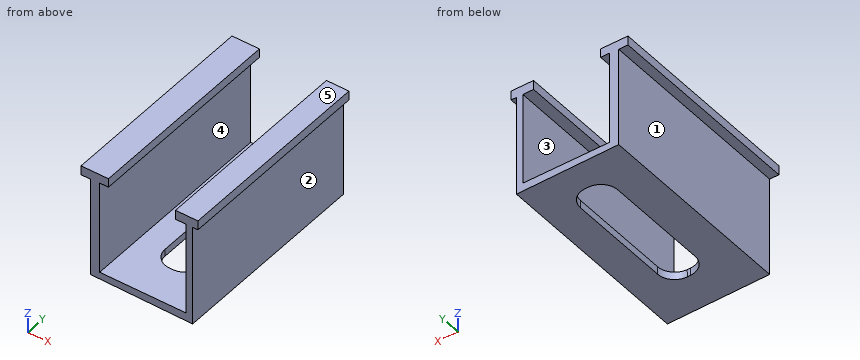
from build123d import *

# Parameters (mm, degrees)
F1_DEPTH = 120
F3_DEPTH = 25
F4_DEPTH = 25


with BuildPart() as f1:
    # F0 (on Front) → F1 (new body)
    with BuildSketch(Plane.XZ):
        Polygon((-31.802535, 29.50009), (-31.802535, 34.680594), (-47.919657, 34.680594), (-47.919657, 29.212285), (-42.451348, 29.212285), (-42.451348, -29.212285), (17.700056, -30.075703), (17.700056, 29.212285), (20.865917, 29.212285), (20.865917, 34.680594), (7.626853, 34.680594), (7.626853, 29.212285), (13.958578, 29.212285), (13.958578, -25.183003), (-36.983039, -25.183003), (-36.983039, 29.50009), align=None)
    extrude(amount=F1_DEPTH)

    # F2 (on face) → F3 (cut)
    with BuildSketch(Plane(origin=(-0.427974, 0, -29.815492), x_dir=(0.999897, 0, -0.014353), z_dir=(-0.014353, 0, -0.999897))):
        with BuildLine():
            Line((-10, 97.833304), (-11.900108, 97.833304))
            ThreePointArc((-11.900108, 97.833304), (-18.971176, 94.904371), (-21.900108, 87.833304))
            Line((-21.900108, 87.833304), (-21.900108, 26.494442))
            ThreePointArc((-21.900108, 26.494442), (-18.971176, 19.423374), (-11.900108, 16.494442))
            Line((-11.900108, 16.494442), (-10, 16.494442))
            ThreePointArc((-10, 16.494442), (-2.928932, 19.423374), (0, 26.494442))
            Line((0, 26.494442), (0, 87.833304))
            ThreePointArc((0, 87.833304), (-2.928932, 94.904371), (-10, 97.833304))
        make_face()
    extrude(amount=F3_DEPTH, mode=Mode.SUBTRACT)

    # F2 (on face) → F4 (cut)
    with BuildSketch(Plane(origin=(-0.427974, 0, -29.815492), x_dir=(0.999897, 0, -0.014353), z_dir=(-0.014353, 0, -0.999897))):
        with BuildLine():
            Line((-10, 97.833304), (-11.900108, 97.833304))
            ThreePointArc((-11.900108, 97.833304), (-18.971176, 94.904371), (-21.900108, 87.833304))
            Line((-21.900108, 87.833304), (-21.900108, 26.494442))
            ThreePointArc((-21.900108, 26.494442), (-18.971176, 19.423374), (-11.900108, 16.494442))
            Line((-11.900108, 16.494442), (-10, 16.494442))
            ThreePointArc((-10, 16.494442), (-2.928932, 19.423374), (0, 26.494442))
            Line((0, 26.494442), (0, 87.833304))
            ThreePointArc((0, 87.833304), (-2.928932, 94.904371), (-10, 97.833304))
        make_face()
    extrude(amount=-F4_DEPTH, mode=Mode.SUBTRACT)


solid = f1.part
Input: part model. Units: mm. Frame: model coordinates. Face numbers are marked on the shaded views. A direction names the side the tool comes from. Coordinates: 2 decimals unless noted, no trailing zeros. Order: outer loops, then holes, each group sorted by start corner. A loop starts at its lowest first (then second) coordinate and runs counter-clockwise, first axis right, second up.
1. Cut plane A-A, the plane z = 14. Return loops of the section in (x, y).
Checked values:
outline: (-42.45, -120) - (-36.98, -120) - (-36.98, 0) - (-42.45, 0) - close; (13.96, -120) - (17.7, -120) - (17.7, 0) - (13.96, 0) - close
2. Cut plane D-D, the plane y = -107. Return loops of the section in (x, z), plus the area to 3 significant figures.
Checked values:
outline: (-47.92, 29.21) - (-42.45, 29.21) - (-42.45, -29.21) - (17.7, -30.08) - (17.7, 29.21) - (20.87, 29.21) - (20.87, 34.68) - (7.63, 34.68) - (7.63, 29.21) - (13.96, 29.21) - (13.96, -25.18) - (-36.98, -25.18) - (-36.98, 29.5) - (-31.8, 29.5) - (-31.8, 34.68) - (-47.92, 34.68) - close
area: 928 mm2
3. Contact query for flat-ended pins moving along their axis: P1, Ø4, axis at x = -21.5, y = -20, coming from the +Z side; P2, Ø1.6, axis at x = -11, z = -27, coming from the +Y side; P3, Ø2.5, axis at x = -44, y = -50, coming from the -Z side; P4, Ø2, axis at y = -47, z = 4, coming from the +X side. Output: stop coordinate, or through.
Checked values:
P1: stops at z = -25.18
P2: stops at y = 0
P3: stops at z = 29.21
P4: stops at x = 17.7
4. Cut plane C-C, the plane x = -34. Return loops of the section in (y, z).
Checked values:
outline: (-120, -29.33) - (0, -29.33) - (0, -25.18) - (-120, -25.18) - close; (-120, 29.5) - (0, 29.5) - (0, 34.68) - (-120, 34.68) - close
5. Access query for the marked faces 4 and 5. Directions: +Z, -Z, +X, -X, +Y, -Y. A direction counts if a zero-diameter tool reaches every point of the face in a straight line with its end or side. Return the directions, or none.
Checked values:
face 4: +Y, -Y
face 5: +Z, +X, -X, +Y, -Y
6. Draft query along X for the marked faces 1, 2 and 3. Return one class per face: +X half, -X half, draft (parallel to the pull), parting line (faces both ways), or undercut.
Checked values:
face 1: -X half
face 2: +X half
face 3: undercut
7. Ray query, line 1 along X through (y, z) = (-16, -1); line 2 along Z through (x, y) = (-41, -49); line 3 along Z through (x, y) = (9, -7). Return the intervals inside material, ascending.
Checked values:
line 1: x = -42.45 to -36.98, 13.96 to 17.7
line 2: z = -29.23 to 34.68
line 3: z = -29.95 to -25.18, 29.21 to 34.68
8. Cut plane B-B, the plane y = -84. Return loops of the section in (x, z), plus the area to 3 significant figures.
Checked values:
outline: (-47.92, 29.21) - (-42.45, 29.21) - (-42.45, -29.21) - (-22.33, -29.5) - (-22.26, -25.18) - (-36.98, -25.18) - (-36.98, 29.5) - (-31.8, 29.5) - (-31.8, 34.68) - (-47.92, 34.68) - close; (-0.43, -29.82) - (17.7, -30.08) - (17.7, 29.21) - (20.87, 29.21) - (20.87, 34.68) - (7.63, 34.68) - (7.63, 29.21) - (13.96, 29.21) - (13.96, -25.18) - (-0.36, -25.18) - close
area: 830 mm2
